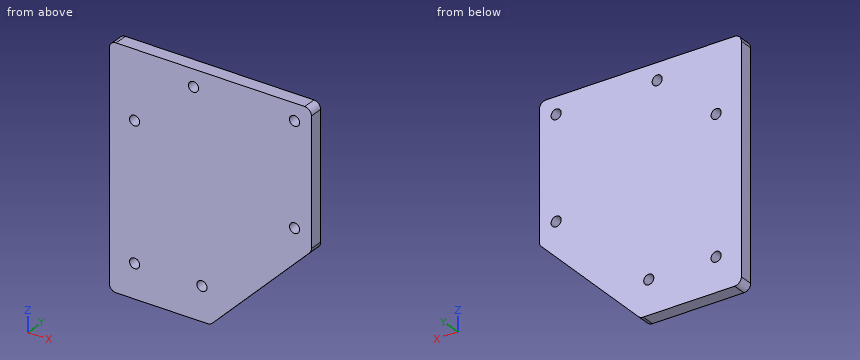
```python
from build123d import *

# Parameters (mm, degrees)
EXTRUDE_1_DEPTH     = 4
SKETCH_2_R          = 1.5
CUT_EXTRUDE_1_DEPTH = 4
FILLET_1_R          = 2
SKETCH_3_R          = 1.5
CUT_EXTRUDE_2_DEPTH = 4
SKETCH_4_R          = 1.5
CUT_EXTRUDE_3_DEPTH = 4
SKETCH_5_R          = 1.5
CUT_EXTRUDE_4_DEPTH = 4
SKETCH_6_R          = 1.5
CUT_EXTRUDE_5_DEPTH = 4


with BuildPart() as part:
    # 草图1 → 凸台-拉伸1 (new body)
    with BuildSketch(Plane(origin=(0, 0, 0), x_dir=(1, 0, 0), z_dir=(0, 1, 0))):
        Polygon((0, 0), (60, 0), (60, 40), (30, 70), (0, 70), align=None)
    extrude(amount=EXTRUDE_1_DEPTH)

    # 草图2 → 切除-拉伸1 (cut)
    with BuildSketch(Plane(origin=(0, 4, 0), x_dir=(1, 0, 0), z_dir=(0, 1, 0))):
        with Locations(Location((7.5, 20, 0), (0, 0, 270))):
            Circle(SKETCH_2_R)
        with Locations(Location((7.5, 60, 0), (0, 0, 270))):
            Circle(SKETCH_2_R)
    extrude(amount=-CUT_EXTRUDE_1_DEPTH, mode=Mode.SUBTRACT)

    # 圆角1
    fillet_1_edges = [part.edges().sort_by_distance(p)[0] for p in [
        (0, 2, -70),
        (30, 2, -70),
        (60, 2, -40),
        (60, 2, 0),
        (0, 2, 0),
    ]]
    fillet(fillet_1_edges, radius=FILLET_1_R)

    # 草图3 → 切除-拉伸2 (cut)
    with BuildSketch(Plane(origin=(0, 4, 0), x_dir=(1, 0, 0), z_dir=(0, 1, 0))):
        with Locations(Location((55, 5, 0), (0, 0, 270))):
            Circle(SKETCH_3_R)
    extrude(amount=-CUT_EXTRUDE_2_DEPTH, mode=Mode.SUBTRACT)

    # 草图4 → 切除-拉伸3 (cut)
    with BuildSketch(Plane(origin=(0, 4, 0), x_dir=(1, 0, 0), z_dir=(0, 1, 0))):
        with Locations(Location((27.5, 60, 0), (0, 0, 270))):
            Circle(SKETCH_4_R)
    extrude(amount=-CUT_EXTRUDE_3_DEPTH, mode=Mode.SUBTRACT)

    # 草图5 → 切除-拉伸4 (cut)
    with BuildSketch(Plane(origin=(0, 4, 0), x_dir=(1, 0, 0), z_dir=(0, 1, 0))):
        with Locations(Location((25, 5, 0), (0, 0, 270))):
            Circle(SKETCH_5_R)
    extrude(amount=-CUT_EXTRUDE_4_DEPTH, mode=Mode.SUBTRACT)

    # 草图6 → 切除-拉伸5 (cut)
    with BuildSketch(Plane(origin=(0, 4, 0), x_dir=(1, 0, 0), z_dir=(0, 1, 0))):
        with Locations(Location((55, 35, 0), (0, 0, 270))):
            Circle(SKETCH_6_R)
    extrude(amount=-CUT_EXTRUDE_5_DEPTH, mode=Mode.SUBTRACT)


solid = part.part
```
Work out the finished part from the listing and answer in its coordinate system (mm). Give positions to 0.01 mm unless a question says otherwise; leave off trailing zeros. Write each loop counter-clockwise with the first axis right and the second up, starting at its lowest first coordinate (ties: lowest second). Pieces come first, ordered by that corner, then holes. Notation, with made-up numbers: (1.25, 69) - (24.25, 69) arc R24 ccw to (24.25, 82) - close; hole circle Ø9 at (16.5, 37.5). An arc over 180 degrees is marked (long way). Use one line per item in the form item = value.
1. A cutting plane is placed at B-B (y = 0.85). Write down the section's boundary in (x, z).
Filled in:
outline = (0, -68) arc R2 ccw to (2, -70) - (29.17, -70) arc R2 ccw to (30.59, -69.41) - (59.41, -40.59) arc R2 ccw to (60, -39.17) - (60, -2) arc R2 ccw to (58, 0) - (2, 0) arc R2 ccw to (0, -2) - close; hole circle Ø3 at (7.5, -60); hole circle Ø3 at (7.5, -20); hole circle Ø3 at (25, -5); hole circle Ø3 at (27.5, -60); hole circle Ø3 at (55, -35); hole circle Ø3 at (55, -5)
2. This flat-tipped pin is pushed along its axis until it touches: pin 1 Ø1.8 at (x, z) = (55, -35) entering from -Y. Where does it stop, or does it pass through?
Filled in:
pin_1 = through
3. Consider L1, parallel to X at y = 2.2, z = -5; L2, parallel to X at y = 1.6, z = -59.5; L3, parallel to X at y = 3.6, z = -20. Determine where each line is inside the solid, lowest interval first.
Filled in:
L1 = 0 to 23.5, 26.5 to 53.5, 56.5 to 60
L2 = 0 to 6.09, 8.91 to 26.09, 28.91 to 40.5
L3 = 0 to 6, 9 to 60
4. A cutting plane is placed at C-C (z = -60). Write down the section's boundary in (x, y), and give its area (3 significant figures).
Filled in:
outline = (0, 0) - (6, 0) - (6, 4) - (0, 4) - close; (9, 0) - (26, 0) - (26, 4) - (9, 4) - close; (29, 0) - (40, 0) - (40, 4) - (29, 4) - close
area = 136 mm^2
5. A cutting plane is placed at D-D (x = 25). Write down the section's boundary in (y, z), and give its area (3 significant figures).
Filled in:
outline = (0, -70) - (4, -70) - (4, -6.5) - (0, -6.5) - close; (0, -3.5) - (4, -3.5) - (4, 0) - (0, 0) - close
area = 268 mm^2
6. A cutting plane is placed at A-A (x = 55). Write down the section's boundary in (y, z).
Filled in:
outline = (0, -45) - (4, -45) - (4, -36.5) - (0, -36.5) - close; (0, -33.5) - (4, -33.5) - (4, -6.5) - (0, -6.5) - close; (0, -3.5) - (4, -3.5) - (4, 0) - (0, 0) - close
